```python
from build123d import *

# Parameters (mm, degrees)
SKETCH1_W           = 20
SKETCH1_H           = 30
SKETCH1_R           = 4
SKETCH1_R_2         = 2.1
BOSS_EXTRUDE1_DEPTH = 10
SKETCH2_R           = 1.15
SKETCH2_R_2         = 2.1
CUT_EXTRUDE1_DEPTH  = 31


with BuildPart() as part:
    # Sketch1 → Boss-Extrude1 (new body)
    with BuildSketch(Plane.XY):
        with Locations((10, 15)):
            Rectangle(SKETCH1_W, SKETCH1_H)
        with Locations((10, 10)):
            Circle(SKETCH1_R, mode=Mode.SUBTRACT)
        with Locations((10, 22)):
            Circle(SKETCH1_R_2, mode=Mode.SUBTRACT)
    extrude(amount=BOSS_EXTRUDE1_DEPTH)

    # Sketch2 → Cut-Extrude1 (cut, through all)
    with BuildSketch(Plane(origin=(0, 30, 0), x_dir=(1, 0, 0), z_dir=(0, 1, 0))):
        with Locations((3, -5)):
            Circle(SKETCH2_R)
        with Locations((17, -5)):
            Circle(SKETCH2_R)
        with Locations((10, -5)):
            Circle(SKETCH2_R_2)
    extrude(amount=-CUT_EXTRUDE1_DEPTH, mode=Mode.SUBTRACT)


solid = part.part
```
Check sheet for the modelled part. Datum: model origin and axes. Units: mm. Coordinates: 2 decimals unless noted, no trailing zeros. Write each loop counter-clockwise with the first axis right and the second up, starting at its lowest first coordinate (ties: lowest second). Pieces come first, ordered by that corner, then holes. Notation, with made-up numbers: (-29, -11.5) - (23, -11.5) arc R16 ccw to (23, 15.5) - close; hole circle Ø7 at (78.25, 62). An arc over 180 degrees is marked (long way). One line per question, with ' | ' between items.
Item 1: Sectioned sample at A-A on y = 10. Record the boundary of the cut face in (x, z).
Determined:
outline: (0, 0) - (6, 0) - (6, 10) - (0, 10) - close; (14, 0) - (20, 0) - (20, 10) - (14, 10) - close; hole circle Ø2.3 at (3, 5); hole circle Ø2.3 at (17, 5)
Item 2: Sectioned sample at C-C on z = 3.5. Record the boundary of the cut face in (x, y).
Determined:
outline: (0, 0) - (8.53, 0) - (8.53, 6.28) arc R4 cw to (8.53, 13.72) - (8.53, 20.5) arc R2.1 cw to (8.53, 23.5) - (8.53, 30) - (0, 30) - close; (11.47, 0) - (20, 0) - (20, 30) - (11.47, 30) - (11.47, 23.5) arc R2.1 cw to (11.47, 20.5) - (11.47, 13.72) arc R4 cw to (11.47, 6.28) - close
Item 3: Gauge pin test, flat end, axial feed: P1, Ø1.4, axis at x = 3, z = 5, coming from the +Y side. Record the tip position at first contact, or that the pin passes through.
Determined:
P1: passes through
Item 4: Mould release check, pull along X, two halves, no side actions. Record for faces 1 (the face through (9.9, 0, 2.7)), 2 (the face through (20, 15, 5)), 3 (the face through (7.9, 3.34, 4.91)), 4 (the face through (0, 15, 5)): pulls with the +X half, pulls with the -X half, needs draft (parallel to the pull), parting line crosses it, or undercut.
Determined:
face 1: needs draft | face 2: pulls with the +X half | face 3: undercut | face 4: pulls with the -X half
Item 5: Thickness scan on line 1 (X direction, y = 24.5, z = 5); line 2 (Y direction, x = 10, z = 2.5); line 3 (Z direction, x = 10, y = 28). Record the ranges inside material, lowest first. Write a range as [from, to].
Determined:
line 1: x = [0, 1.85], [4.15, 7.9], [12.1, 15.85], [18.15, 20] | line 2: y = [0, 6], [14, 19.9], [24.1, 30] | line 3: z = [0, 2.9], [7.1, 10]
Item 6: Sectioned sample at D-D on y = 5.5. Record the boundary of the cut face in (x, z).
Determined:
outline: (0, 0) - (20, 0) - (20, 10) - (0, 10) - close; hole circle Ø2.3 at (3, 5); hole circle Ø4.2 at (10, 5); hole circle Ø2.3 at (17, 5)
Item 7: Sectioned sample at B-B on x = 17. Record the boundary of the cut face in (y, z).
Determined:
outline: (0, 0) - (30, 0) - (30, 3.85) - (0, 3.85) - close; (0, 6.15) - (30, 6.15) - (30, 10) - (0, 10) - close
